Part model, mm, in its own coordinate system. Face numbers are marked on the shaded views. A direction names the side the tool comes from. Coordinates: 2 decimals unless noted, no trailing zeros. Loops run counter-clockwise (first coordinate to the right, second up) from the corner with the lowest first, then second, coordinate; pieces in that order, holes last. Notation, with made-up numbers: (9, 30) -> (65, 30) arc R13 ccw to (65, 52) -> close; hole circle Ø1 at (4.25, -24.5). An arc over 180 degrees is marked (long way). One line per question, with ' | ' between items. Start each with the question number.
1) Cut at C-C (z = -10). List the corners of the cut face in (x, y).
2) Cut at A-A (x = 0). List the corners of the cut face in (y, z), plus the area to 3 significant figures.
3) Probe L1, parallel to Z at x = 3.5, y = -7.25; L2, parallel to Z at x = -5.5, y = 2; L3, parallel to X at y = 0.75, z = -6.5. List the from-to ranges inside material, lowest first. Write a range as from..to.
4) Drop flat-ended pins along their axis: pin 1 (3.5 mm diameter, centred on x = -1, y = 3, fed in from -Z); pin 2 (8 mm diameter, centred on x = -1, z = -18, fed in from -Y); pin 3 (10 mm diameter, centred on y = -4, z = -14.5, fed in from +X). Give the stop position or say it passes through.
5) 3-axis set-ups, long thin cutter, end or side, ignore diameter. For the marked faces 1 and 2: which of +Z, -Z, +X, -X, +Y, -Y reach the whole face in a straight line?
Autodesk Inventor part; units mm, degrees
ref_plane "YZ Plane" through (0, 0, 0) normal (1, 0, 0) x (0, 1, 0)
ref_plane "XZ Plane" through (0, 0, 0) normal (0, 1, 0) x (-1, 0, 0)
ref_plane "XY Plane" through (0, 0, 0) normal (0, 0, 1) x (1, 0, 0)
sketch "Esboço1" plane through (0, 0, 0) normal (0, 0, 1) x (1, 0, 0)
  circle A0 centre (0, 0) radius 3.5
  circle A1 centre (0, 0) radius 3
  point P0 (0, 0)
  dimension "d0" = 6
extrude "Extrusão1" add sketch "Esboço1" against normal blind 25 contours A1
fillet "Arredondamento1" radius 3 1 edges at (-3, 0, -25)
sketch "Esboço2" plane through (0, 0, 0) normal (0, 0, 1) x (1, 0, 0)
  circle A0 centre (0, 0) radius 3
  point P0 (0, 0)
extrude "Extrusão2" add sketch "Esboço2" along normal blind 3
sketch "Esboço3" plane through (0, 0, 3) normal (0, 0, 1) x (1, 0, 0)
  circle A0 centre (0, 0) radius 3
  circle A1 centre (0, 0) radius 6
  point P0 (0, 0)
  dimension "d6" = 12
extrude "Extrusão3" add sketch "Esboço3" along normal blind 1.5 contours A0 | A1
sketch "Esboço4" plane through (0, 0, 4.5) normal (0, 0, 1) x (1, 0, 0)
  circle A0 centre (0, 0) radius 9
  dimension "d9" = 18
extrude "Extrusão4" add sketch "Esboço4" along normal blind 5
chamfer "Chanfro1" distance 0.5 angle 45 2 edges at (-9, 0, 9.5) (-9, 0, 4.5)
properties part number "Pino de Liberação Valvula Alivio de Pressão"
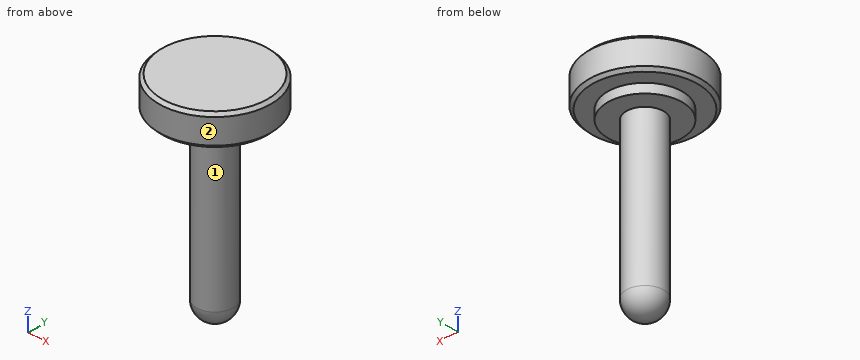
Reported:
1) outline: circle Ø6 at (0, 0)
2) outline: (-9, 5) -> (-8.5, 4.5) -> (-6, 4.5) -> (-6, 3) -> (-3, 3) -> (-3, -22) arc R3 ccw to (3, -22) -> (3, 3) -> (6, 3) -> (6, 4.5) -> (8.5, 4.5) -> (9, 5) -> (9, 9) -> (8.5, 9.5) -> (-8.5, 9.5) -> (-9, 9) -> close | area: 272 mm²
3) L1: z = 4.5..9.5 | L2: z = 3..9.5 | L3: x = -2.9..2.9
4) pin 1: stops at z = -24.65 | pin 2: stops at y = -3 | pin 3: stops at x = 3
5) face 1: -Z | face 2: +Z, -Z
